Source: CAD feature listing. Evaluate the final solid. Frame: model axes, mm. A direction names the side the tool comes from. Give positions to 0.01 mm unless a question says otherwise; leave off trailing zeros. Write each loop counter-clockwise with the first axis right and the second up, starting at its lowest first coordinate (ties: lowest second). Pieces come first, ordered by that corner, then holes. Notation, with made-up numbers: M 25,1.25 L 81,1.25 A10 ccw 81,16.25 Z; hole C 61.5,15 d7. An arc over 180 degrees is marked long. Use CSV: the item, a comma, the result in double quotes. Start each with the question number.
from build123d import *

# Parameters (mm, degrees)
SKETCH1_R           = 1.5
BOSS_EXTRUDE1_DEPTH = 1.12
SKETCH2_W           = 6
SKETCH2_H           = 9.83
BOSS_EXTRUDE2_DEPTH = 5.55
BOSS_EXTRUDE3_DEPTH = 9.83
SKETCH4_R           = 6.45
BOSS_EXTRUDE4_DEPTH = 12.2


with BuildPart() as part:
    # Sketch1 → Boss-Extrude1 (new body)
    with BuildSketch(Plane(origin=(0, 0, 0), x_dir=(1, 0, 0), z_dir=(0, 1, 0))):
        with BuildLine():
            Line((3.5, 0), (26.5, 0))
            ThreePointArc((26.5, 0), (28.974873734, 1.025126266), (30, 3.5))
            Line((30, 3.5), (30, 18.5))
            ThreePointArc((30, 18.5), (28.974873734, 20.974873734), (26.5, 22))
            Line((26.5, 22), (3.5, 22))
            ThreePointArc((3.5, 22), (1.025126266, 20.974873734), (0, 18.5))
            Line((0, 18.5), (0, 3.5))
            ThreePointArc((0, 3.5), (1.025126266, 1.025126266), (3.5, 0))
        make_face()
        with Locations(Location((26.5, 18.5, 0), (0, 0, 270))):
            Circle(SKETCH1_R, mode=Mode.SUBTRACT)
        with Locations(Location((26.5, 3.5, 0), (0, 0, 270))):
            Circle(SKETCH1_R, mode=Mode.SUBTRACT)
    extrude(amount=BOSS_EXTRUDE1_DEPTH)

    # Sketch2 → Boss-Extrude2 (add)
    with BuildSketch(Plane(origin=(0, 1.12, 0), x_dir=(1, 0, 0), z_dir=(0, 1, 0))):
        with Locations((3, 11)):
            Rectangle(SKETCH2_W, SKETCH2_H)
    extrude(amount=BOSS_EXTRUDE2_DEPTH)

    # Sketch3 → Boss-Extrude3 (add)
    with BuildSketch(Plane.XY.offset(-6.085)):
        Polygon((0, 1.12), (7.54, 1.12), (6, 6.67), (0, 6.67), align=None)
    extrude(amount=-BOSS_EXTRUDE3_DEPTH)

    # Sketch4 → Boss-Extrude4 (add)
    with BuildSketch(Plane(origin=(0, 1.12, 0), x_dir=(1, 0, 0), z_dir=(0, 1, 0))):
        with Locations(Location((17.76, 11, 0), (0, 0, 270))):
            Circle(SKETCH4_R)
    extrude(amount=BOSS_EXTRUDE4_DEPTH)


solid = part.part
1. Section C-C on z = -5.75. Return loops of the section in (x, y).
2. Pull-direction query (X, two-part tool) for faces 6 (the flat face through (15, 0, -11)), 7 (the flat face through (0, 3, -11)), 8 (the cylindrical face through (29, 0.55, -20.95)), 9 (the cylindrical face through (27.51, 0.55, -19.61)); classes: released by +X, released by -X, zero draft, split by the parting line, or undercut.
3. Line query: probe 1 along X at (y, z) = (0.4, -3.5); probe 2 along Z at (x, y) = (3.75, 6.5) (3 decimals); probe 3 along Y at (x, z) = (2.25, -21). Output: solid intervals per line, ascending.
4. Section A-A on x = 17.76. Return loops of the section in (y, z).
5. First-contact query: pin 1 (5 mm diameter, centred on x = 4, z = -9, fed in from +Y); pin 2 (1.5 mm diameter, centred on y = 7, z = -14.5, fed in from +X); pin 3 (4 mm diameter, centred on y = 3, z = -2.5, fed in from -X). Flat tips, straight axial feed; report the tip coordinate or a pass-through.
6. Section D-D on y = 9. Return loops of the section in (x, z), then the cut area to 3 significant figures.
7. Section B-B on y = 4. Return loops of the section in (x, z) (3 decimals), then the cut area to 3 significant figures.
8. Access query for faces 1 (the flat face through (4, 4, -6.085)), 2 (the cylindrical face through (12.04, 7.13, -8.02)), 3 (the flat face through (6.78, 3.86, -10.93)), 4 (the flat face through (3, 6.67, -11)), 5 (the flat face through (4, 4, -15.915)). Directions: +Z, -Z, +X, -X, +Y, -Y. A direction counts if a zero-diameter tool reaches every point of the face in a straight line with its end or side. Return the directions, or none.
Resolved:
1,outline,"M 0,0 L 30,0 L 30,1.12 L 21.51,1.12 L 21.51,13.32 L 14.01,13.32 L 14.01,1.12 L 0,1.12 Z"
2,face 6,"zero draft"
2,face 7,"released by -X"
2,face 8,"released by +X"
2,face 9,"undercut"
3,probe 1,"x = 0 to 25, 28 to 30"
3,probe 2,"z = -15.915 to -6.085"
3,probe 3,"y = 0 to 1.12"
4,outline,"M 0,-22 L 1.12,-22 L 1.12,-17.45 L 13.32,-17.45 L 13.32,-4.55 L 1.12,-4.55 L 1.12,0 L 0,0 Z"
5,pin 1,"stops at y = 6.67"
5,pin 2,"stops at x = 23.59"
5,pin 3,"stops at x = 0.01"
6,outline,"C 17.76,-11 d12.9"
6,area,"131 mm2"
7,outline,"M 0,-15.915 L 6.741,-15.915 L 6.741,-6.085 L 0,-6.085 Z; C 17.76,-11 d12.9"
7,area,"197 mm2"
8,face 1,"+Z, -X, +Y"
8,face 2,"+Y"
8,face 3,"+Z, -Z, +Y"
8,face 4,"+Z, -Z, -X, +Y"
8,face 5,"-Z, -X, +Y"
